Geometry check sheet. Reference: the model listing, model coordinates, mm. Face numbers are marked on the shaded views. A direction names the side the tool comes from. Round coordinates to 2 decimals unless told otherwise and drop trailing zeros. Loops run counter-clockwise (first coordinate to the right, second up) from the corner with the lowest first, then second, coordinate; pieces in that order, holes last. Notation, with made-up numbers: (-3.5, -25.75) - (8.5, -25.75) arc R10 cw to (8.5, -21.75) - close; hole circle Ø6 at (12, 82.5). An arc over 180 degrees is marked (long way). Write item = value, one per line.
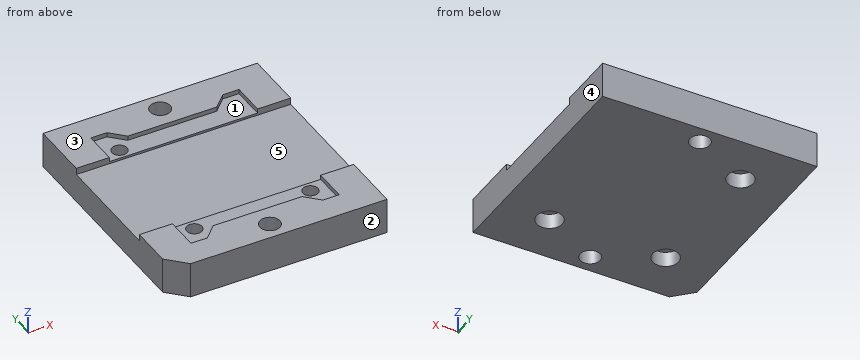
Autodesk Inventor part; units mm, degrees
ref_plane "YZ Plane" through (0, 0, 0) normal (1, 0, 0) x (0, 1, 0)
ref_plane "XZ Plane" through (0, 0, 0) normal (0, 1, 0) x (-1, 0, 0)
ref_plane "XY Plane" through (0, 0, 0) normal (0, 0, 1) x (1, 0, 0)
sketch "Sketch1" plane through (0, 0, 0) normal (0, 0, 1) x (1, 0, 0)
  line L0 (-24, 26) -> (24, 26)
  line L1 (24, 26) -> (24, -26)
  line L2 (24, -26) -> (-24, -26)
  line L3 (-24, -26) -> (-24, 26)
  line L4 (-24, 26) -> (24, -26) construction
  line L5 (24, 26) -> (-24, -26) construction
  point P0 (0, 0)
  dimension "d2" = 48
  dimension "d3" = 52
extrude "Extrusion1" add sketch "Sketch1" along normal blind 8
sketch "Sketch2" plane through (0, 0, 8) normal (0, 0, 1) x (1, 0, 0)
  line L0 (0, 22) -> (0, -22) construction
  point P0 (0, 0)
  point P1 (0, 0)
  dimension "d4" = 44
hole "Hole1" at (0, 22, 8) at (0, -22, 8) direction (0, 0, -1) diameter 4.5 depth 20
sketch "Sketch3" plane through (0, 0, 8) normal (0, 0, 1) x (1, 0, 0)
  line L0 (13, -20) -> (16.5, -20)
  line L1 (10, -17) -> (-10, -17)
  line L2 (13, 20) -> (16.5, 20)
  line L3 (-10, 17) -> (10, 17)
  line L4 (-13, 20) -> (-16.5, 20)
  line L5 (-13, 20) -> (-10, 17)
  line L6 (10, 17) -> (13, 20)
  line L7 (13, -20) -> (10, -17)
  line L8 (-10, -17) -> (-13, -20)
  line L9 (-13, -20) -> (-16.5, -20)
  circle A0 centre (0, 22) radius 2.25 construction
  circle A1 centre (0, -22) radius 2.25 construction
  line L10 (-24, -26) -> (24, -26) construction
  line L11 (24, -26) -> (24, 26) construction
  line L12 (24, 26) -> (-24, 26) construction
  line L13 (-24, 26) -> (-24, -26) construction
  line L14 (16.5, -20) -> (16.5, 20)
  line L15 (-16.5, 20) -> (-16.5, -20)
  point P0 (0, 0)
extrude "Extrusion2" cut sketch "Sketch3" against normal blind 0.9
sketch "Sketch4" plane through (0, 0, 0) normal (0, 0, -1) x (-1, 0, 0)
  line L0 (-13, -15) -> (13, -15) construction
  line L1 (13, -15) -> (13, 15) construction
  line L2 (13, 15) -> (-13, 15) construction
  line L3 (-13, 15) -> (-13, -15) construction
  line L4 (-13, -15) -> (13, 15) construction
  line L5 (13, -15) -> (-13, 15) construction
  point P0 (0, 0)
  dimension "d16" = 26
  dimension "d17" = 30
hole "Hole2" at (-13, 15, 0) at (-13, -15, 0) at (13, -15, 0) direction (0, 0, 1) diameter 3.4 end through all counterbore diameter 5.8 counterbore depth 3.4
chamfer "Chamfer1" distance 4 angle 45 1 edges at (-24, -26, 4)
thicken "Thicken1" operation cut thickness 0.1 both sides no extend neighbours no toward (0, 1, 0) faces at (-14.1667, 20, 7.7) (-11, 18, 7.7) (3.3333, 17, 7.4) (12, 19, 7.7) (15.3333, 20, 7.7) (11, -18, 7.7) (14.1667, -20, 7.7) (-3.3333, -17, 7.7) (-15.3333, -20, 7.7) (-12, -19, 7.7) (3.3333, 5.6667, 7.1) (16.5, -6.6667, 7.7) (-16.5, 6.6667, 7.7)
sketch "Sketch5" plane through (0, 0, 8) normal (0, 0, 1) x (1, 0, 0)
  line L0 (24, 12.65) -> (-24, 12.65)
  line L1 (-24, 12.65) -> (-24, -12.65)
  line L2 (-24, -12.65) -> (24, -12.65)
  line L3 (24, -12.65) -> (24, 12.65)
  line L4 (24, 12.65) -> (-24, -12.65) construction
  line L5 (-24, 12.65) -> (24, -12.65) construction
  line L6 (24, -26) -> (24, 26) construction
  point P0 (0, 0)
  dimension "d28" = 25.3
extrude "Extrusion3" cut sketch "Sketch5" against normal blind 1.5
properties part number "ChamberMount_c"
(1) Section check C-C (z = 4.25). Enter the section's corners in (x, y).
Answers follow:
outline = (-24, -22) - (-20, -26) - (24, -26) - (24, 26) - (-24, 26) - close; hole circle Ø3.4 at (-13, -15); hole circle Ø3.4 at (-13, 15); hole circle Ø4.5 at (0, -22); hole circle Ø4.5 at (0, 22); hole circle Ø3.4 at (13, -15)
(2) Mould release check, pull along Y, two halves, no side actions. Record for the marked faces 1, 2 and 3: pulls with the +Y half, pulls with the -Y half, needs draft (parallel to the pull), parting line crosses it, or undercut.
Answers follow:
face_1 = undercut
face_2 = pulls with the -Y half
face_3 = needs draft
(3) Set-up check for the marked faces 4 and 5: record each of +Z, -Z, +X, -X, +Y, -Y from which the full face is reachable in a straight line by a thin tool's end or side.
Answers follow:
face_4 = +Z, -Z, +X, +Y, -Y
face_5 = +Z, +X, -X
(4) Section check B-B (x = 0). Enter the section's corners in (y, z).
Answers follow:
outline = (-26, 0) - (-24.25, 0) - (-24.25, 8) - (-26, 8) - close; (-19.75, 0) - (19.75, 0) - (19.75, 8) - (17.1, 8) - (17.1, 7) - (12.65, 7) - (12.65, 6.5) - (-12.65, 6.5) - (-12.65, 7) - (-17.1, 7) - (-17.1, 8) - (-19.75, 8) - close; (24.25, 0) - (26, 0) - (26, 8) - (24.25, 8) - close
(5) Gauge pin test, flat ends, axial feed: pin 1 (1.7 mm diameter, centred on x = -14, y = 15, fed in from -Z); pin 2 (5 mm diameter, centred on x = -7.5, y = -14.5, fed in from +Z). Record the tip position at first contact, or that the pin passes through.
Answers follow:
pin_1 = 3.4
pin_2 = 7
(6) Section check D-D (y = -15). Enter the section's corners in (x, z), then the cut area to 3 significant figures.
Answers follow:
outline = (-24, 0) - (-15.9, 0) - (-15.9, 3.4) - (-14.7, 3.4) - (-14.7, 7) - (-16.6, 7) - (-16.6, 8) - (-24, 8) - close; (-11.3, 3.4) - (-10.1, 3.4) - (-10.1, 0) - (10.1, 0) - (10.1, 3.4) - (11.3, 3.4) - (11.3, 7) - (-11.3, 7) - close; (14.7, 3.4) - (15.9, 3.4) - (15.9, 0) - (24, 0) - (24, 8) - (16.6, 8) - (16.6, 7) - (14.7, 7) - close
area = 287 mm²
(7) Scan lines: L1, parallel to X at y = -15, z = 2.4; L2, parallel to Y at x = -13, z = 4.4; L3, parallel to Y at x = 0, z = 6. Record each from-to range of solid material in increasing order. Write a range as [from, to].
Answers follow:
L1 = [-24, -15.9], [-10.1, 10.1], [15.9, 24]
L2 = [-26, -16.7], [-13.3, 13.3], [16.7, 26]
L3 = [-26, -24.25], [-19.75, 19.75], [24.25, 26]
(8) Section check A-A (y = 15). Enter the section's corners in (x, z).
Answers follow:
outline = (-24, 0) - (-15.9, 0) - (-15.9, 3.4) - (-14.7, 3.4) - (-14.7, 7) - (-16.6, 7) - (-16.6, 8) - (-24, 8) - close; (-11.3, 3.4) - (-10.1, 3.4) - (-10.1, 0) - (24, 0) - (24, 8) - (16.6, 8) - (16.6, 7) - (-11.3, 7) - close
